Here's the drawing with two shaded views (mm, measured from the low corner). I have some questions. A direction names the side the tool comes from. Round coordinates to 2 decimals unless told otherwise and drop trailing zeros. Order: outer loops, then holes, each group sorted by start corner. A loop starts at its lowest first (then second) coordinate and runs counter-clockwise, first axis right, second up.
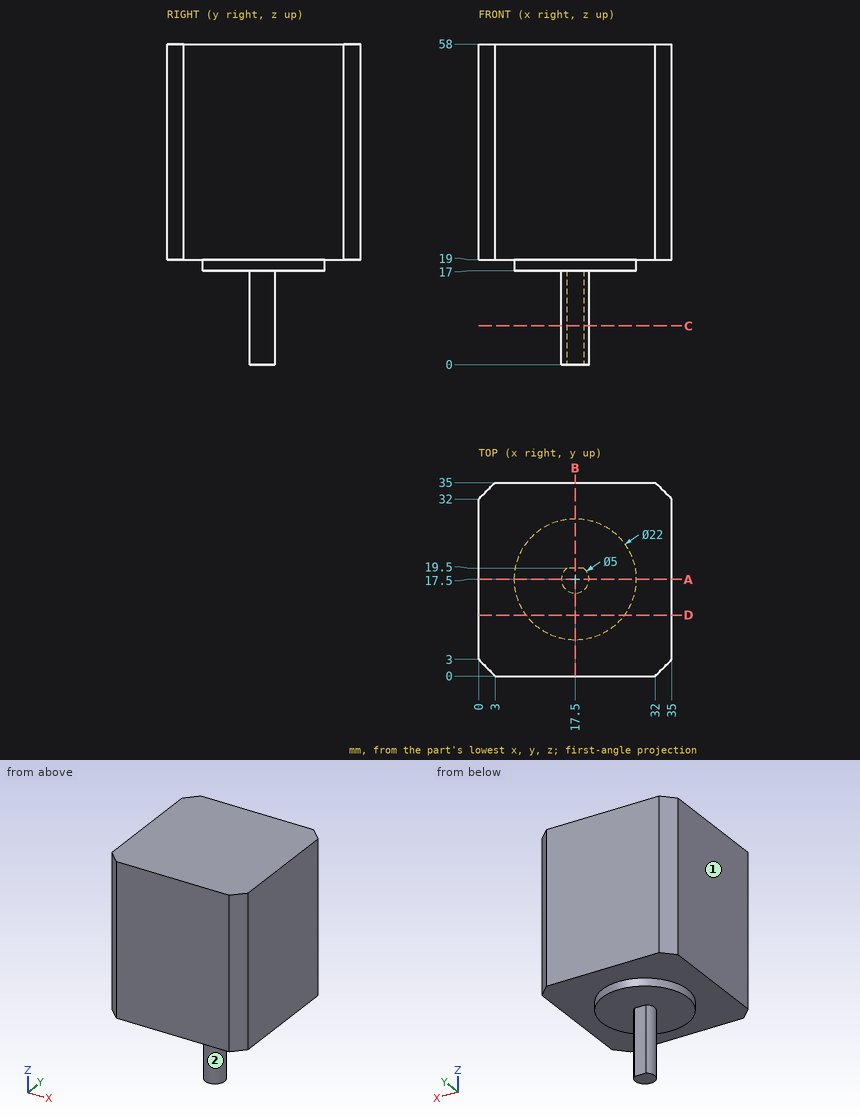
Q1. Imagine slicing it at D-D, the plane y = 11. Please give me the cut outline in (x, z).
Q2. Imagine slicing it at A-A, the plane y = 17.5. Please give me the cut outline in (x, z).
Q3. For the marked faces 1 and 2, which set-ups out of +Z, -Z, +X, -X, +Y, -Y let a thin tool reach every point of the face, with its end or its side?
Q4. Imagine slicing it at B-B, the plane x = 17.5. Please give me the cut outline in (y, z), then the cut area to 3 significant figures.
Q5. For P1, Ø6.5, axis at x = 21.5, y = 16.5, coming from the -Z side; P2, Ø10, axis at x = 21.5, z = 10.5, coming from the +Y side; P3, Ø3, axis at x = 26, y = 6, coming from the -Z side, each with a flat end and sliding along its axis, tell me the tip position at first contact or that it passes through.
Q6. Imagine slicing it at C-C, the plane z = 7. Please give me the cut outline in (x, y), then the cut area to 3 significant figures.
Q7. I need wall thicknesses on L1, parallel to Z at x = 26, y = 9.5; L2, parallel to Z at x = 14.5, y = 27; L3, parallel to Y at x = 15.5, z = 5.5. Which ranges of each line are inside material? Lowest first, please.
Filled in:
1. outline: (0, 19) - (8.63, 19) - (8.63, 17) - (26.37, 17) - (26.37, 19) - (35, 19) - (35, 58) - (0, 58) - close
2. outline: (0, 19) - (6.5, 19) - (6.5, 17) - (15, 17) - (15, 0) - (20, 0) - (20, 17) - (28.5, 17) - (28.5, 19) - (35, 19) - (35, 58) - (0, 58) - close
3. face 1: +Z, -Z, -X, +Y, -Y
3. face 2: -Z
4. outline: (0, 19) - (6.5, 19) - (6.5, 17) - (15, 17) - (15, 0) - (19.5, 0) - (19.5, 17) - (28.5, 17) - (28.5, 19) - (35, 19) - (35, 58) - (0, 58) - close
4. area: 1,490 mm2
5. P1: stops at z = 0
5. P2: stops at y = 19.5
5. P3: stops at z = 19
6. outline: (16, 19.5) arc R2.5 ccw (long way) to (19, 19.5) - close
6. area: 18.6 mm2
7. L1: z = 19 to 58
7. L2: z = 17 to 58
7. L3: y = 16 to 19
